Autodesk Inventor part; units mm, degrees
ref_plane "YZ Plane" through (0, 0, 0) normal (1, 0, 0) x (0, 1, 0)
ref_plane "XZ Plane" through (0, 0, 0) normal (0, 1, 0) x (-1, 0, 0)
ref_plane "XY Plane" through (0, 0, 0) normal (0, 0, 1) x (1, 0, 0)
sketch "Sketch1" plane through (0, 0, 0) normal (0, 1, 0) x (-1, 0, 0)
  line L0 (0, 0) -> (-2.5, 0)
  line L1 (-2.5, 0) -> (-2.5, 14)
  line L2 (-2.5, 14) -> (-1.3, 14)
  line L3 (-1.3, 14) -> (-1.3, 19)
  line L4 (-1.3, 19) -> (0, 19)
  line L5 (0, 19) -> (0, 0)
  dimension "d1" = 5
  dimension "d2" = 14
  dimension "d3" = 2.6
  dimension "d4" = 5
revolve "Revolution1" add sketch "Sketch1" angle 360 about axis through (0, 0, 19) along (0, 0, -1)
sketch "Sketch2" plane through (0, 0, 0) normal (0, 0, -1) x (-1, 0, 0)
  line L0 (-2.5, -0.5) -> (2.5, -0.5)
  line L1 (2.5, -0.5) -> (2.5, 0.5)
  line L2 (2.5, 0.5) -> (-2.5, 0.5)
  line L3 (-2.5, 0.5) -> (-2.5, -0.5)
  line L4 (-2.5, -0.5) -> (2.5, 0.5) construction
  line L5 (2.5, -0.5) -> (-2.5, 0.5) construction
  circle A0 centre (0, 0) radius 2.5
  dimension "d6" = 1
extrude "Extrusion1" cut sketch "Sketch2" against normal blind 1 contours L3 A0 L0 | A0 L2 L0 | L3 L2 A0 | A0 L1 L0 | A0 L2 L1
hole "Hole1" at (0, 0, 0) direction (0, 0, 1) diameter 2.1129 depth 5
thread "Thread1"
chamfer "Chamfer1" distance 0.3 angle 45 7 edges at (-2.5, 0, 14) (0, 2.5, 0) (0, -2.5, 0) (0, -1.0564, 0) (-0.5421, 0.9067, 0) (0.5421, 0.9067, 0) (-1.3, 0, 19)
properties part number "BRU-2614S" material "Stainless Steel AISI 304"
Can you work these out from the model? Positions are in its coordinate system, mm. A direction names the side the tool comes from. Coordinates: 2 decimals unless noted, no trailing zeros. Write each loop counter-clockwise with the first axis right and the second up, starting at its lowest first coordinate (ties: lowest second). Pieces come first, ordered by that corner, then holes.
Q1. If we mould it in two halves opening along X, with no side actions, what happens to faces 1 (the face through (-1.047, -0.138, 2.683)), 2 (the face through (-0.54, -2.44, 7.09)), 3 (the face through (-1.7, 0.5, 0.5))? For each: +X half, -X half, draft (parallel to the pull), parting line (faces both ways), or undercut.
Results found:
face 1: undercut
face 2: parting line
face 3: draft
Q2. Imagine slicing it at C-C, the plane z = 2.75. List the corners of the cut face in (x, y) for me.
Results found:
outline: circle Ø5 at (0, 0); hole circle Ø2.11 at (0, 0)
Q3. For P1, Ø0.8, axis at x = 2, y = 0, coming from the -Z side; P2, Ø1, axis at x = -0.5, y = -0.5, coming from the -Z side; P3, Ø3, axis at x = -1.5, z = 16, coming from the +Y side, each with a flat end and sliding along its axis, tell me the tip position at first contact or that it passes through.
Results found:
P1: stops at z = 1
P2: stops at z = 0.15
P3: stops at y = 1.3
Q4. Which directions (+Z, -Z, +X, -X, +Y, -Y) give clear straight access to the entire face, cutting with the end or side of a thin tool? Please do faces 4 (the face through (0, 2, 0)), 5 (the face through (0, 0, 5)), 6 (the face through (-2, 0, 1)), 7 (the face through (-0.17, 1.29, 16.38)).
Results found:
face 4: -Z, +X, -X, +Y, -Y
face 5: -Z
face 6: -Z, +X, -X
face 7: +Z
Q5. Please list where these lines run through material, in increasing order: L1, parallel to X at y = 0, z = 1.75; L2, parallel to Z at x = 1, y = 1.2.
Results found:
L1: x = -2.5 to -1.06, 1.06 to 2.5
L2: z = 0 to 14
Q6. Imagine slicing it at A-A, the plane y = 0. List the corners of the cut face in (x, z) for me, plus the area to 3 significant figures.
Results found:
outline: (-2.5, 1) - (-1.06, 1) - (-1.06, 5) - (1.06, 5) - (1.06, 1) - (2.5, 1) - (2.5, 13.7) - (2.2, 14) - (1.3, 14) - (1.3, 18.7) - (1, 19) - (-1, 19) - (-1.3, 18.7) - (-1.3, 14) - (-2.2, 14) - (-2.5, 13.7) - close
area: 69.4 mm2
Q7. Imagine slicing it at B-B, the plane x = 0. List the corners of the cut face in (y, z) for me, plus the area to 3 significant figures.
Results found:
outline: (-2.5, 0.3) - (-2.2, 0) - (-1.36, 0) - (-1.06, 0.3) - (-1.06, 5) - (1.06, 5) - (1.06, 0.3) - (1.36, 0) - (2.2, 0) - (2.5, 0.3) - (2.5, 13.7) - (2.2, 14) - (1.3, 14) - (1.3, 18.7) - (1, 19) - (-1, 19) - (-1.3, 18.7) - (-1.3, 14) - (-2.2, 14) - (-2.5, 13.7) - close
area: 72.1 mm2
Q8. Imagine slicing it at D-D, the plane z = 6. List the corners of the cut face in (x, y) for me, plus the area to 3 significant figures.
Results found:
outline: circle Ø5 at (0, 0)
area: 19.6 mm2
